Read the model definition and answer for the solid it produces. Units are mm, in the model's axes. Face numbers are marked on the shaded views. A direction names the side the tool comes from. Round coordinates to 2 decimals unless told otherwise and drop trailing zeros. Order: outer loops, then holes, each group sorted by start corner. A loop starts at its lowest first (then second) coordinate and runs counter-clockwise, first axis right, second up. Notation, with made-up numbers: (-23.5, 76.25) - (7.5, 76.25) arc R17 cw to (7.5, 84.25) - close; hole circle Ø10 at (16.5, 46). An arc over 180 degrees is marked (long way). Put each result on its own line as item: value. Start each with the question number.
Q1. Section B-B on y = -179 is taken. Give the vertices of the cut face in (x, z), then the cut area to 3 significant figures.
Q2. Section A-A on y = 80.5 is taken. Give the vertices of the cut face in (x, z), then the cut area to 3 significant figures.
Q3. Each of these flat-tipped pins is pushed along its axis until it touches: pin 1 Ø10 at (x, z) = (-44, -2.5) entering from +Y; pin 2 Ø10 at (y, z) = (-168.5, 31.5) entering from -X; pin 3 Ø12 at (y, z) = (138, -22) entering from +X. Where does it stop, or does it pass through?
Q4. Which of the six approach directions +Z, -Z, +X, -X, +Y, -Y give full straight-line access (tool end or side, diameter ignored) to the marked faces 1 and 2?
Q5. Find the intervals of material crossed by line 1 along Y through (x, z) = (11.5, 47); line 2 along Z through (x, y) = (-6, 67.5); line 3 along Z through (x, y) = (37, 191.5), in increasing order. Write a range as from..to.
from build123d import *

# Parameters (mm, degrees)
F0_R     = 57.15
F1_DEPTH = 228.6
F2_R     = 44.45
F3_W     = 317.5
F3_H     = 76.2
F4_DEPTH = 57.151


with BuildPart() as f1:
    # F0 (on Front) → F1 (new body, symmetric)
    with BuildSketch(Plane.XZ):
        Circle(F0_R)
    extrude(amount=F1_DEPTH, both=True)

    # F2
    f2_edges = [f1.edges().sort_by_distance(p)[0] for p in [
        (-57.15, -228.6, 0),
        (-57.15, 228.6, 0),
    ]]
    fillet(f2_edges, radius=F2_R)

    # F3 (on Right) → F4 (cut, through all)
    with BuildSketch(Plane.YZ):
        with Locations((0, 38.1)):
            Rectangle(F3_W, F3_H)
    extrude(amount=F4_DEPTH, mode=Mode.SUBTRACT)


solid = f1.part
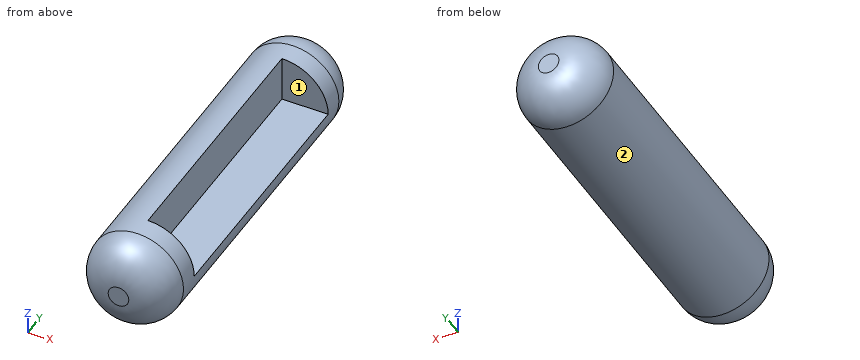
Findings:
1. outline: circle Ø114.3 at (0, 0)
1. area: 10,300 mm2
2. outline: (0, 0) - (0, 57.15) arc R57.15 ccw (long way) to (57.15, 0) - close
2. area: 7,700 mm2
3. pin 1: y = 219.93
3. pin 2: x = -50.63
3. pin 3: x = 54.86
4. face 1: +Z, +X
4. face 2: +Y, -Y
5. line 1: -210.65..-158.75, 158.75..210.65
5. line 2: -56.83..56.83
5. line 3: -42.75..42.75
